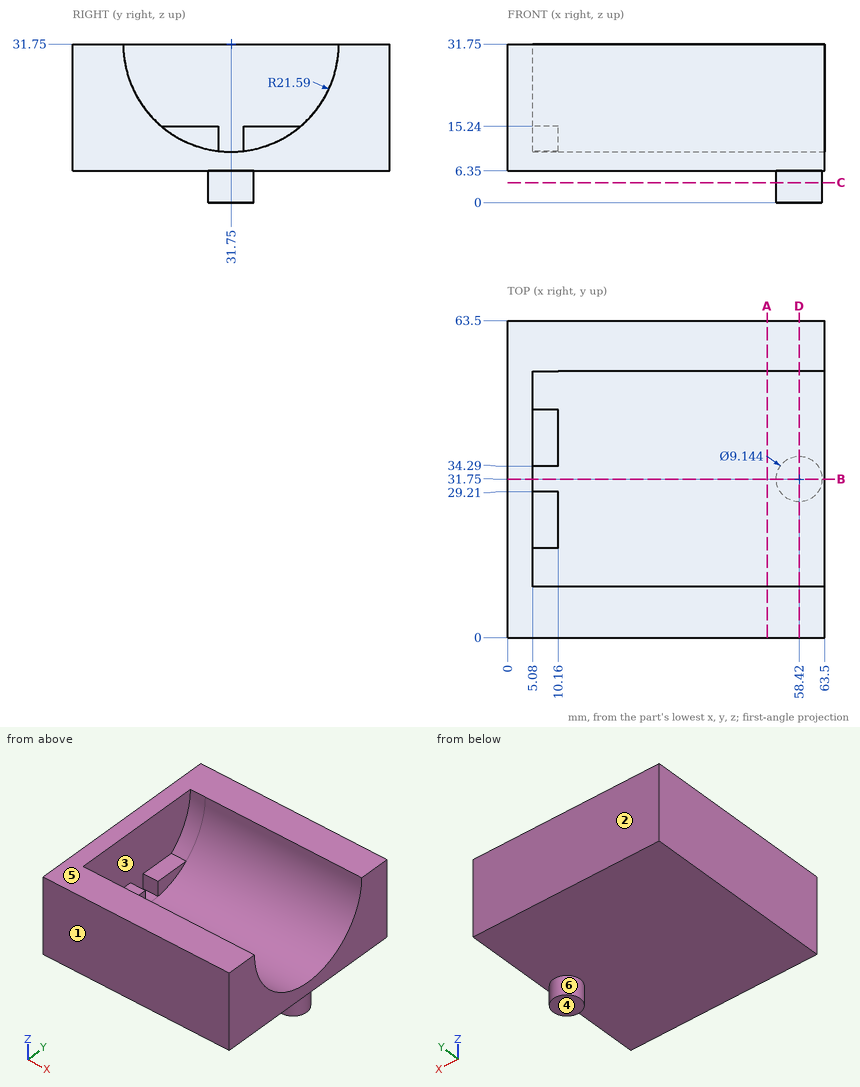
Geometry check sheet. Reference: drawing and pictorial views, mm from the part's lowest x, y, z. A direction names the side the tool comes from. Coordinates: 2 decimals unless noted, no trailing zeros. Write each loop counter-clockwise with the first axis right and the second up, starting at its lowest first coordinate (ties: lowest second). Pieces come first, ordered by that corner, then holes. Notation, with made-up numbers: (42, 40.25) -> (53, 40.25) arc R15 cw to (53, 44.25) -> close; hole circle Ø10 at (29, 54.25). An arc over 180 degrees is marked (long way). Use a Markdown table: item, result.
1. Go/stop test with flat-tipped pins: pin 1 Ø4 at (x, y) = (18.5, 43.5) entering from +Z; pin 2 Ø3 at (x, y) = (16.5, 43.5) entering from -Z; pin 3 Ø2.5 at (y, z) = (39, 13) entering from +X. Record where each tip stops, or that it passes through.
Reported:
| item | result |
|---|---|
| pin 1 | stops at z = 15.1 |
| pin 2 | stops at z = 6.35 |
| pin 3 | stops at x = 10.16 |
2. Release check for a two-part mould opening along Y. For the marked faces 1, 2, 3 and 4 record: pulls with the +Y half, pulls with the -Y half, needs draft (parallel to the pull), parting line crosses it, or undercut.
Reported:
| item | result |
|---|---|
| face 1 | pulls with the -Y half |
| face 2 | pulls with the +Y half |
| face 3 | undercut |
| face 4 | needs draft |
3. Tool access check on the marked faces 5 and 6. Record the directions out of +Z, -Z, +X, -X, +Y, -Y that give a thin tool (end or side, any length) a straight path to the whole face; none if there is none.
Reported:
| item | result |
|---|---|
| face 5 | +Z, +X, -X, +Y, -Y |
| face 6 | -Z |
4. Sectioned sample at B-B (y = 31.75). Enter the section's corners in (x, z), plus the area to 3 significant figures.
Reported:
| item | result |
|---|---|
| outline | (0, 6.35) -> (53.85, 6.35) -> (53.85, 0) -> (62.99, 0) -> (62.99, 6.35) -> (63.5, 6.35) -> (63.5, 10.16) -> (5.08, 10.16) -> (5.08, 31.75) -> (0, 31.75) -> close |
| area | 410 mm2 |
5. Scan lines: line 1 along X through (y, z) = (37, 26); line 2 along Z through (x, y) = (13.5, 6.5); line 3 along Y through (x, z) = (40, 16). Record each from-to range of solid material in increasing order.
Reported:
| item | result |
|---|---|
| line 1 | x = 0 to 5.08 |
| line 2 | z = 6.35 to 31.75 |
| line 3 | y = 0 to 16.98, 46.52 to 63.5 |
6. Sectioned sample at D-D (x = 58.42). Enter the section's corners in (y, z), plus the area to 3 significant figures.
Reported:
| item | result |
|---|---|
| outline | (0, 6.35) -> (27.18, 6.35) -> (27.18, 0) -> (36.32, 0) -> (36.32, 6.35) -> (63.5, 6.35) -> (63.5, 31.75) -> (53.34, 31.75) arc R21.59 cw to (10.16, 31.75) -> (0, 31.75) -> close |
| area | 939 mm2 |
7. Sectioned sample at A-A (x = 52). Enter the section's corners in (y, z), plus the area to 3 significant figures.
Reported:
| item | result |
|---|---|
| outline | (0, 6.35) -> (63.5, 6.35) -> (63.5, 31.75) -> (53.34, 31.75) arc R21.59 cw to (10.16, 31.75) -> (0, 31.75) -> close |
| area | 881 mm2 |
8. Sectioned sample at C-C (z = 4). Enter the section's corners in (x, y), plus the area to 3 significant figures.
Reported:
| item | result |
|---|---|
| outline | circle Ø9.14 at (58.42, 31.75) |
| area | 65.7 mm2 |
